The listing builds one solid part. Answer for the finished solid, in the listing's coordinates (mm). A direction names the side the tool comes from. Round coordinates to 2 decimals unless told otherwise and drop trailing zeros. Order: outer loops, then holes, each group sorted by start corner. A loop starts at its lowest first (then second) coordinate and runs counter-clockwise, first axis right, second up. Notation, with made-up numbers: (39.25, -28.5) - (85.25, -28.5) arc R8 ccw to (85.25, -23.5) - close; hole circle Ø4 at (12, 56.25). An arc over 180 degrees is marked (long way). Write item = value, one per line.
Solid Edge part; units mm, degrees
sketch "Sketch1" plane through (0, 0, 0) normal (0, 0, 1) x (1, 0, 0)
  line L0 (90, 67.5) -> (-90, 67.5)
  line L1 (-90, 67.5) -> (-90, -67.5)
  line L2 (-90, -67.5) -> (90, -67.5)
  line L3 (90, -67.5) -> (90, 67.5)
  circle A0 centre (-78.5, 57.5) radius 1.6
  circle A1 centre (78.5, 57.5) radius 1.6
  circle A2 centre (78.5, -57.5) radius 1.6
  line L4 (-65, 44) -> (-15, 44)
  line L5 (-15, 41) -> (-65, 41)
  arc A3 (-15, 44) -> (-15, 41) centre (-15, 42.5) cw
  arc A4 (-65, 41) -> (-65, 44) centre (-65, 42.5) cw
  line L6 (-65.2368, 24) -> (-15.2368, 24)
  line L7 (-15.2368, 21) -> (-65.2368, 21)
  arc A5 (-15.2368, 24) -> (-15.2368, 21) centre (-15.2368, 22.5) cw
  arc A6 (-65.2368, 21) -> (-65.2368, 24) centre (-65.2368, 22.5) cw
  line L8 (-65.2368, 4) -> (-15.2368, 4)
  line L9 (-15.2368, 1) -> (-65.2368, 1)
  arc A7 (-15.2368, 4) -> (-15.2368, 1) centre (-15.2368, 2.5) cw
  arc A8 (-65.2368, 1) -> (-65.2368, 4) centre (-65.2368, 2.5) cw
  line L10 (-65.2368, -16) -> (-15.2368, -16)
  line L11 (-15.2368, -19) -> (-65.2368, -19)
  arc A9 (-15.2368, -16) -> (-15.2368, -19) centre (-15.2368, -17.5) cw
  arc A10 (-65.2368, -19) -> (-65.2368, -16) centre (-65.2368, -17.5) cw
  line L12 (-65.2368, -36) -> (-15.2368, -36)
  line L13 (-15.2368, -39) -> (-65.2368, -39)
  arc A11 (-15.2368, -36) -> (-15.2368, -39) centre (-15.2368, -37.5) cw
  arc A12 (-65.2368, -39) -> (-65.2368, -36) centre (-65.2368, -37.5) cw
  line L14 (14.9672, -36) -> (64.9672, -36)
  line L15 (64.9672, -39) -> (14.9672, -39)
  arc A13 (64.9672, -36) -> (64.9672, -39) centre (64.9672, -37.5) cw
  arc A14 (14.9672, -39) -> (14.9672, -36) centre (14.9672, -37.5) cw
  line L16 (64.9672, -16) -> (14.9672, -16)
  line L17 (14.9672, -19) -> (64.9672, -19)
  arc A15 (14.9672, -19) -> (14.9672, -16) centre (14.9672, -17.5) cw
  arc A16 (64.9672, -16) -> (64.9672, -19) centre (64.9672, -17.5) cw
  line L18 (64.9672, 4) -> (14.9672, 4)
  line L19 (14.9672, 1) -> (64.9672, 1)
  arc A17 (14.9672, 1) -> (14.9672, 4) centre (14.9672, 2.5) cw
  arc A18 (64.9672, 4) -> (64.9672, 1) centre (64.9672, 2.5) cw
  line L20 (64.9672, 24) -> (14.9672, 24)
  line L21 (14.9672, 21) -> (64.9672, 21)
  arc A19 (14.9672, 21) -> (14.9672, 24) centre (14.9672, 22.5) cw
  arc A20 (64.9672, 24) -> (64.9672, 21) centre (64.9672, 22.5) cw
  line L22 (15, 41) -> (65, 41)
  line L23 (65, 44) -> (15, 44)
  arc A21 (65, 44) -> (65, 41) centre (65, 42.5) cw
  arc A22 (15, 41) -> (15, 44) centre (15, 42.5) cw
  circle A23 centre (-78.5, -57.5) radius 1.6
extrude "Protrusion1" add sketch "Sketch1" along normal blind 3.5
sketch "Sketch2" plane through (0, 0, 0) normal (0, 0, -1) x (-1, 0, 0)
  line L0 (-75.6, 55.8257) -> (-75.6, 59.1743)
  line L1 (-75.6, 59.1743) -> (-78.5, 60.8486)
  line L2 (-78.5, 60.8486) -> (-81.4, 59.1743)
  line L3 (-81.4, 59.1743) -> (-81.4, 55.8257)
  line L4 (-81.4, 55.8257) -> (-78.5, 54.1514)
  line L5 (-78.5, 54.1514) -> (-75.6, 55.8257)
  line L6 (-78.5, -60.8486) -> (-75.6, -59.1743)
  line L7 (-75.6, -59.1743) -> (-75.6, -55.8257)
  line L8 (-75.6, -55.8257) -> (-78.5, -54.1514)
  line L9 (-78.5, -54.1514) -> (-81.4, -55.8257)
  line L10 (-81.4, -55.8257) -> (-81.4, -59.1743)
  line L11 (-81.4, -59.1743) -> (-78.5, -60.8486)
  line L12 (81.4, 55.8257) -> (81.4, 59.1743)
  line L13 (81.4, 59.1743) -> (78.5, 60.8486)
  line L14 (78.5, 60.8486) -> (75.6, 59.1743)
  line L15 (75.6, 59.1743) -> (75.6, 55.8257)
  line L16 (75.6, 55.8257) -> (78.5, 54.1514)
  line L17 (78.5, 54.1514) -> (81.4, 55.8257)
  line L18 (75.6, -55.8257) -> (75.6, -59.1743)
  line L19 (75.6, -59.1743) -> (78.5, -60.8486)
  line L20 (78.5, -60.8486) -> (81.4, -59.1743)
  line L21 (81.4, -59.1743) -> (81.4, -55.8257)
  line L22 (81.4, -55.8257) -> (78.5, -54.1514)
  line L23 (78.5, -54.1514) -> (75.6, -55.8257)
extrude "ExtrudedCutout_1" cut sketch "Sketch2" against normal blind 4
sketch "Sketch3" plane through (0, 0, 3.5) normal (0, 0, 1) x (1, 0, 0)
  line L0 (-82.5, 61.5) -> (82.5, 61.5)
  line L1 (82.5, 61.5) -> (82.5, -61.5)
  line L2 (-82.5, -61.5) -> (82.5, -61.5)
  line L3 (-82.5, -61.5) -> (-82.5, 61.5)
  line L4 (-73.5, 52.5) -> (73.5, 52.5)
  line L5 (73.5, -52.5) -> (73.5, 52.5)
  line L6 (73.5, -52.5) -> (-73.5, -52.5)
  line L7 (-73.5, -52.5) -> (-73.5, 52.5)
extrude "ExtrudedProtrusion_2" add sketch "Sketch3" along normal blind 6.8
sketch "Sketch4" plane through (0, 0, 10.3) normal (0, 0, 1) x (1, 0, 0)
  circle A0 centre (-78.5, 57.5) radius 1.6
  circle A1 centre (-78.5, -57.5) radius 1.6
  circle A2 centre (78.5, -57.5) radius 1.6
  circle A3 centre (78.5, 57.5) radius 1.6
extrude "Cutout1" cut sketch "Sketch4" against normal through all
sketch "Sketch5" plane through (82.5, 0, 8) normal (1, 0, 0) x (0, 1, 0)
  line L0 (-2.5, -4.5) -> (-2.5, 2.3)
  line L1 (-2.5, 2.3) -> (47.5, 2.3)
  line L2 (47.5, 2.3) -> (47.5, -4.5)
  line L3 (47.5, -4.5) -> (-2.5, -4.5)
extrude "Cutout2" cut sketch "Sketch5" against normal up to next
sketch "Sketch6" plane through (0, 0, 3.5) normal (0, 0, 1) x (1, 0, 0)
  circle A0 centre (-45, 12.5) radius 1.65
  circle A1 centre (-45, -29.5) radius 1.65
  circle A2 centre (45, -29.5) radius 1.65
  circle A3 centre (45, 12.5) radius 1.65
extrude "Cutout3" cut sketch "Sketch6" against normal up to next
fillet "Round1" radius 5 4 edges at (90, 67.5, 1.75) (-90, 67.5, 1.75) (-90, -67.5, 1.75) (90, -67.5, 1.75)
sketch "Sketch7" plane through (0, 0, 3.5) normal (0, 0, 1) x (1, 0, 0)
  line L0 (90, 9.5) -> (73.5, 9.5)
  line L1 (73.5, 9.5) -> (73.5, 47.5)
  line L2 (73.5, 47.5) -> (90, 47.5)
  line L3 (90, 47.5) -> (90, 9.5)
extrude "Cutout4" cut sketch "Sketch7" against normal up to next
fillet "Round_2" radius 3 2 edges at (90, 47.5, 1.75) (90, 9.5, 1.75)
Q1. Determine the mould class of faces 4 (the face through (-41, -36, 2)), 5 (the face through (0, -54, 10.3)), 6 (the face through (82.5, -32, 7)) for opening direction X: released by +X, released by -X, zero draft, split by the parting line, or undercut.
Model answer:
face_4 = undercut
face_5 = zero draft
face_6 = released by +X
Q2. Flat-ended cylindrical pins translate along their axes: P1, Ø1, axis at x = 8, z = 8.5, coming from the +Y side; P2, Ø3, axis at x = -53, y = -36, coming from the +Z side; P3, Ø2, axis at y = -18, z = 6, coming from the -X side. Find the tip coordinate at first contact, or state that the pin passes through.
Model answer:
P1 = 61.5
P2 = 3.5
P3 = -82.5
Q3. Section C-C on x = -8 is taken. Determine the outline of the cut face in (y, z).
Model answer:
outline = (-67.5, 0) - (67.5, 0) - (67.5, 3.5) - (61.5, 3.5) - (61.5, 10.3) - (52.5, 10.3) - (52.5, 3.5) - (-52.5, 3.5) - (-52.5, 10.3) - (-61.5, 10.3) - (-61.5, 3.5) - (-67.5, 3.5) - close
Q4. Section B-B on z = 6 is taken. Determine the outline of the cut face in (x, y), then the cut area to 3 significant figures.
Model answer:
outline = (-82.5, -61.5) - (82.5, -61.5) - (82.5, -2.5) - (73.5, -2.5) - (73.5, -52.5) - (-73.5, -52.5) - (-73.5, 52.5) - (73.5, 52.5) - (73.5, 47.5) - (82.5, 47.5) - (82.5, 61.5) - (-82.5, 61.5) - close; hole circle Ø3.2 at (-78.5, -57.5); hole circle Ø3.2 at (-78.5, 57.5); hole circle Ø3.2 at (78.5, -57.5); hole circle Ø3.2 at (78.5, 57.5)
area = 4,380 mm^2
Q5. For faces 1 (the face through (40, 4, 2)), 2 (the face through (-82.5, -1, 7)), 3 (the face through (78, -2.5, 7)), determine the directions among +Z, -Z, +X, -X, +Y, -Y from which every point of the face is accessible in a straight line to the end or side of a thin tool.
Model answer:
face_1 = +Z, -Z
face_2 = +Z, -X, +Y, -Y
face_3 = +Z, +X
Q6. Find the intervals of material crossed by line 1 (Y direction, x = 21, z = 0.75); line 2 (X direction, y = -47, z = 6); line 3 (Y direction, x = -69.5, z = 9), in increasing order. Write a range as from..to.
Model answer:
line_1 = -67.5..-39, -36..-19, -16..1, 4..21, 24..41, 44..67.5
line_2 = -82.5..-73.5, 73.5..82.5
line_3 = -61.5..-52.5, 52.5..61.5
Q7. Section A-A on x = 27 is taken. Count the separate pieces of the cut face and the enclosed holes in it, then the cut area to 3 significant figures.
Model answer:
separate_pieces = 6
enclosed_holes = 0
area = 542 mm^2
